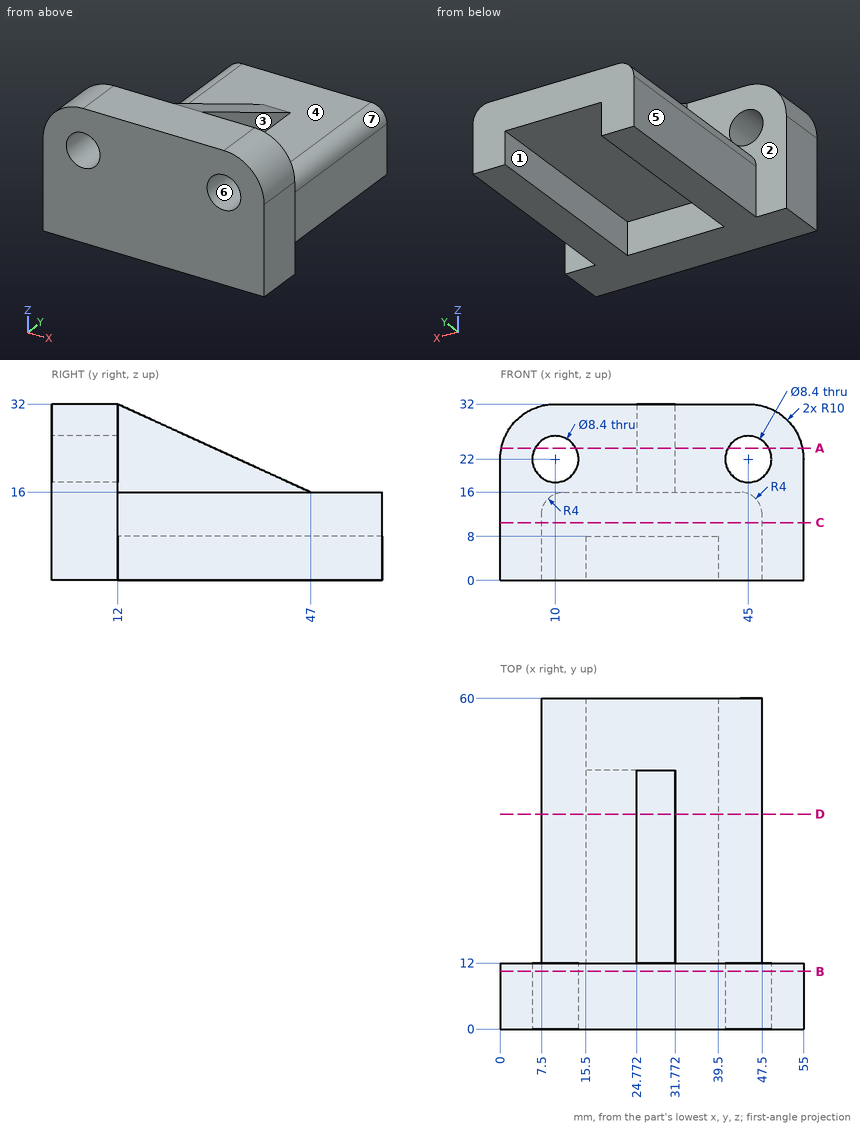
Input: dimensioned drawing with shaded views. Units: mm. Origin: part minimum x, y, z. A direction names the side the tool comes from. Round coordinates to 2 decimals unless told otherwise and drop trailing zeros. Loops run counter-clockwise (first coordinate to the right, second up) from the corner with the lowest first, then second, coordinate; pieces in that order, holes last. Notation, with made-up numbers: (48.25, 38.5) -> (62.25, 38.5) arc R20 cw to (62.25, 76.5) -> close; hole circle Ø5 at (37.5, 43). An arc over 180 degrees is marked (long way). Answer as a JSON object with one key per item and string values. Group by question number.
1) Section query B-B on y = 10.5. Output: boundary loops of the cut face in (x, z).
2) Section query A-A on z = 24. Output: boundary loops of the cut face in (x, y).
3) Reachability of the marked faces 1, 2, 3 and 4 from +Z, -Z, +X, -X, +Y, -Y: full face, straight path, thin tool, end or side. Return the list, or none.
4) Pin query (flat end, axial travel): pin 1 (13 mm diameter, centred on y = 42, z = 6.5, fed in from -X); pin 2 (9.5 mm diameter, centred on x = 28, y = 45, fed in from +Z) (1 decimal); pin 3 (5 mm diameter, centred on y = 9.5, z = 20, fed in from -X); pin 4 (2 mm diameter, centred on y = 25, z = 15.5, fed in from +X). Return the tip coordinate at first contact, or that it passes through.
5) Section query C-C on z = 10.5. Output: boundary loops of the cut face in (x, y).
6) Ray query, L1, parallel to X at y = 24.5, z = 6.5; L2, parallel to Z at x = 45, y = 7; L3, parallel to Y at x = 21.5, z = 18.5. Return the intervals inside material, ascending.
7) Section query D-D on y = 39. Output: boundary loops of the cut face in (x, z).
8) Draft query along Z for the marked faces 5, 6 and 7. Return one class per face: +Z half, -Z half, draft (parallel to the pull), parting line (faces both ways), or undercut.
Reply:
{
 "1": {"outline": "(0, 0) -> (55, 0) -> (55, 22) arc R10 ccw to (45, 32) -> (10, 32) arc R10 ccw to (0, 22) -> close; hole circle Ø8.4 at (10, 22); hole circle Ø8.4 at (45, 22)"},
 "2": {"outline": "(0.2, 0) -> (6.31, 0) -> (6.31, 12) -> (0.2, 12) -> close; (13.69, 0) -> (41.31, 0) -> (41.31, 12) -> (31.77, 12) -> (31.77, 29.5) -> (24.77, 29.5) -> (24.77, 12) -> (13.69, 12) -> close; (48.69, 0) -> (54.8, 0) -> (54.8, 12) -> (48.69, 12) -> close"},
 "3": {"face 1": "-Z, +Y", "face 2": "+Z, -X, +Y", "face 3": "+Z, +X, +Y", "face 4": "+Z, +Y"},
 "4": {"pin 1": "stops at x = 7.5", "pin 2": "stops at z = 19.1", "pin 3": "stops at x = 0", "pin 4": "stops at x = 46.62"},
 "5": {"outline": "(0, 0) -> (55, 0) -> (55, 12) -> (47.5, 12) -> (47.5, 60) -> (7.5, 60) -> (7.5, 12) -> (0, 12) -> close"},
 "6": {"L1": "x = 7.5 to 15.5, 39.5 to 47.5", "L2": "z = 0 to 17.8, 26.2 to 32", "L3": "y = 0 to 12"},
 "7": {"outline": "(7.5, 0) -> (15.5, 0) -> (15.5, 8) -> (39.5, 8) -> (39.5, 0) -> (47.5, 0) -> (47.5, 12) arc R4 ccw to (43.5, 16) -> (31.77, 16) -> (31.77, 19.66) -> (24.77, 19.66) -> (24.77, 16) -> (11.5, 16) arc R4 ccw to (7.5, 12) -> close"},
 "8": {"face 5": "draft", "face 6": "undercut", "face 7": "+Z half"}
}
